Geometry: final body of the model. Coordinates: model frame, mm. A direction names the side the tool comes from. Give positions to 0.01 mm unless a question says otherwise; leave off trailing zeros. Loops run counter-clockwise (first coordinate to the right, second up) from the corner with the lowest first, then second, coordinate; pieces in that order, holes last.
1. Draft query along X for faces 1 (the face through (39.015, 0.66, 0.364)), 2 (the face through (-68.985, 0.66, 0.364)), 3 (the face through (14.505, 63.704, 15.154)), 4 (the face through (-18, 19, 26)). Return one class per face: +X half, -X half, draft (parallel to the pull), parting line (faces both ways), or undercut.
2. Section C-C, the plane z = -3. Output: boundary loops of the cut face in (x, y).
3. Access query for faces 5 (the face through (-24.72, 38.51, -2.08)), 6 (the face through (87.99, 0.75, 0.36)), 7 (the face through (-62.032, 99.675, 9.238)). Directions: +Z, -Z, +X, -X, +Y, -Y. A direction counts if a zero-diameter tool reaches every point of the face in a straight line with its end or side. Return the directions, or none.
4. Material intervals for line 1 along Y through (x, z) = (-54, 0); line 2 along X through (y, z) = (13, -10); line 3 along X through (y, z) = (12.5, -21), sorted ascending.
5. Section A-A, the plane y = 0. Output: boundary loops of the cut face in (x, z), then the cut area to 3 significant figures.
6. Section D-D, the plane x = 47. Output: boundary loops of the cut face in (y, z), then the cut area to 3 significant figures.
7. Section B-B, the plane x = -60.5. Output: boundary loops of the cut face in (y, z).
8. First-contact query: P1, Ø4, axis at x = -56, z = -1, coming from the +Y side; P2, Ø17, axis at y = 48, z = 1, coming from the -X side; P3, Ø2, axis at x = 9.5, z = -6.5, coming from the +Y side; P4, Ø2, axis at x = 66.5, y = 3, coming from the +Z side. Flat tips, straight axial feed; report the tip coordinate or a pass-through.
from build123d import *

# Parameters (mm, degrees)
BOSS_EXTRUDE1_DEPTH = 26
SKETCH2_R           = 15
CUT_EXTRUDE1_DEPTH  = 108.721864076
SKETCH3_R           = 25
SKETCH3_R_2         = 9
BOSS_EXTRUDE2_DEPTH = 34
BOSS_EXTRUDE3_DEPTH = 34
FILLET1_R           = 15
BOSS_EXTRUDE4_DEPTH = 22


with BuildPart() as part:
    # Sketch1 → Boss-Extrude1 (new, symmetric)
    with BuildSketch(Plane.XY):
        with BuildLine():
            Line((-54, 34), (54, 34))
            ThreePointArc((54, 34), (88, 0), (54, -34))
            Line((54, -34), (-54, -34))
            ThreePointArc((-54, -34), (-88, 0), (-54, 34))
        make_face()
    extrude(amount=BOSS_EXTRUDE1_DEPTH, both=True)

    # Sketch2 → Cut-Extrude1 (cut, through all)
    with BuildSketch(Plane.XY.offset(26)):
        with Locations((54, 0)):
            Circle(SKETCH2_R)
        with Locations((-54, 0)):
            Circle(SKETCH2_R)
    extrude(amount=-CUT_EXTRUDE1_DEPTH, mode=Mode.SUBTRACT)



with BuildPart() as body_2:
    # Sketch3 → Boss-Extrude2 (new body)
    with BuildSketch(Plane.XY.offset(26)):
        with Locations((-54, 76)):
            Circle(SKETCH3_R)
        with Locations((-54, 76)):
            Circle(SKETCH3_R_2, mode=Mode.SUBTRACT)
    extrude(amount=-BOSS_EXTRUDE2_DEPTH)


with BuildPart() as part_1:
    add(part.part)

    add(body_2.part)  # Boss-Extrude3 merges body 2
    # Sketch4 → Boss-Extrude3 (add)
    with BuildSketch(Plane.XY.offset(26)):
        with BuildLine():
            Line((-79, 76), (-79, 23.043437244))
            ThreePointArc((-79, 23.043437244), (-67.647767834, 31.140623519), (-54, 34))
            Line((-54, 34), (-29, 34))
            Line((-29, 34), (-29, 76))
            ThreePointArc((-29, 76), (-54, 51), (-79, 76))
        make_face()
    extrude(amount=-BOSS_EXTRUDE3_DEPTH)

    # Fillet1
    fillet1_edges = [part_1.edges().sort_by_distance(p)[0] for p in [
        (-29, 34, 9),
    ]]
    fillet(fillet1_edges, radius=FILLET1_R)

    # Sketch5 → Boss-Extrude4 (add)
    with BuildSketch(Plane.XY.offset(26)):
        with BuildLine():
            Line((-41.03946331, 97.378131086), (71.626329898, 29.074258276))
            ThreePointArc((71.626329898, 29.074258276), (63.150825608, 32.745417858), (54, 34))
            Line((54, 34), (-14, 34))
            ThreePointArc((-14, 34), (-24.606601718, 38.393398282), (-29, 49))
            Line((-29, 49), (-29, 76))
            ThreePointArc((-29, 76), (-32.216825102, 88.26757072), (-41.03946331, 97.378131086))
        make_face()
    extrude(amount=-BOSS_EXTRUDE4_DEPTH)


solid = part_1.part
Answers below:
1. face 1: undercut
1. face 2: undercut
1. face 3: +X half
1. face 4: draft
2. outline: (-79, 23.04) arc R34 ccw to (-54, -34) - (54, -34) arc R34 ccw to (54, 34) - (-14, 34) arc R15 cw to (-29, 49) - (-29, 76) arc R25 ccw to (-79, 76) - close; hole circle Ø30 at (-54, 0); hole circle Ø18 at (-54, 76); hole circle Ø30 at (54, 0)
3. face 5: -Z, +X, +Y
3. face 6: -Z, +X
3. face 7: -Z, +Y
4. line 1: y = -34 to -15, 15 to 67, 85 to 101
4. line 2: x = -85.42 to -61.48, -46.52 to 46.52, 61.48 to 85.42
4. line 3: x = -85.62 to -62.29, -45.71 to 45.71, 62.29 to 85.62
5. outline: (-88, -26) - (-69, -26) - (-69, 26) - (-88, 26) - close; (-39, -26) - (39, -26) - (39, 26) - (-39, 26) - close; (69, -26) - (88, -26) - (88, 26) - (69, 26) - close
5. area: 6,030 mm2
6. outline: (-34, -26) - (-13.27, -26) - (-13.27, 26) - (-34, 26) - close; (13.27, -26) - (34, -26) - (34, 4) - (44, 4) - (44, 26) - (13.27, 26) - close
6. area: 2,380 mm2
7. outline: (-33.37, -26) - (-13.52, -26) - (-13.52, 26) - (-33.37, 26) - close; (13.52, -26) - (33.37, -26) - (33.37, -8) - (69.78, -8) - (69.78, 26) - (13.52, 26) - close; (82.22, -8) - (100.14, -8) - (100.14, 26) - (82.22, 26) - close
8. P1: stops at y = 101
8. P2: stops at x = -79
8. P3: stops at y = 34
8. P4: passes through
